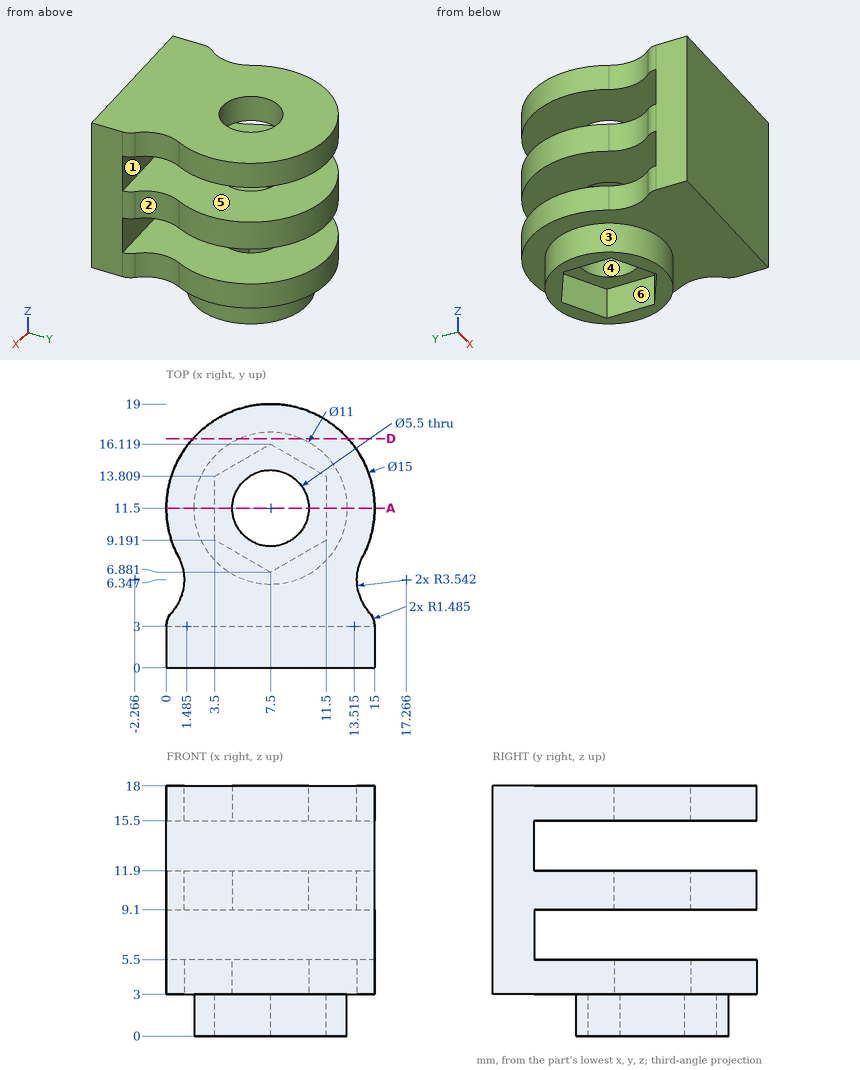
Part print with two shaded views. Sizes in mm from the minimum x, y, z corner. A direction names the side the tool comes from. Coordinates: 2 decimals unless noted, no trailing zeros. Write each loop counter-clockwise with the first axis right and the second up, starting at its lowest first coordinate (ties: lowest second). Pieces come first, ordered by that corner, then holes. Notation, with made-up numbers: M -9,20.25 L 42,20.25 A28 cw 42,56.25 Z; hole C 33.5,-16.5 d6. An arc over 180 degrees is marked long. Return JSON: item names as keys, results as strings.
Item 1: Probe line 1 (Z direction, x = 9, y = 7); line 2 (Z direction, x = 11.25, y = 11); line 3 (Y direction, x = 5.5, z = 5.25) (1 decimal). List the from-to ranges inside material, lowest first. Write a range as from..to.
Findings below:
{"line 1": "z = 0..5.5, 9.1..11.9, 15.5..18", "line 2": "z = 3..5.5, 9.1..11.9, 15.5..18", "line 3": "y = 0..9.6, 13.4..18.7"}
Item 2: Drop flat-ended pins along their axis: pin 1 Ø1.1 at (x, z) = (7, 13.5) entering from +Y; pin 2 Ø1.5 at (y, z) = (11.5, 1.5) entering from +X; pin 3 Ø4 at (y, z) = (8, 3) entering from -X. Give the stop position or say it passes through.
Findings below:
{"pin 1": "stops at y = 3", "pin 2": "stops at x = 13", "pin 3": "stops at x = 0.15"}
Item 3: Slice it at D-D, the plane y = 16.5. Write the cut outline in (x, z).
Findings below:
{"outline": "M 1.91,3 L 5.21,3 L 5.21,0 L 9.79,0 L 9.79,3 L 13.09,3 L 13.09,5.5 L 1.91,5.5 Z; M 1.91,9.1 L 13.09,9.1 L 13.09,11.9 L 1.91,11.9 Z; M 1.91,15.5 L 13.09,15.5 L 13.09,18 L 1.91,18 Z"}
Item 4: Which spindle directions (+Z, -Z, +X, -X, +Y, -Y) get a long thin tool onto all of the face, cutting with end or side? Do the marked faces 4, 5 and 6. Say none if no direction does.
Findings below:
{"face 4": "+Z, -Z", "face 5": "+X, -X, +Y", "face 6": "-Z"}
Item 5: Slice it at A-A, the plane y = 11.5. State how many separate pieces and enclosed holes the cut face has.
Findings below:
{"separate pieces": "6", "enclosed holes": "0"}
Item 6: Two-plate mould, pull along Y, no slides. Class the marked faces 1, 2 and 3: +Y half, -Y half, draft (parallel to the pull), parting line (faces both ways), or undercut.
Findings below:
{"face 1": "+Y half", "face 2": "undercut", "face 3": "parting line"}
